from build123d import *

# Parameters (mm, degrees)
ESBO_O1_W                = 40
ESBO_O1_H                = 50
ESBO_O1_R                = 2
ESBO_O1_H_2              = 20
RESSALTO_EXTRUS_O1_DEPTH = 6
FILETE1_R                = 10


with BuildPart() as part:
    # Esboço1 → Ressalto-extrusão1 (new body)
    # profile 1 of 2: a face of its own
    with BuildSketch(Plane.XY):
        with Locations((20, 25)):
            Rectangle(ESBO_O1_W, ESBO_O1_H)
        with Locations((30, 10)):
            Circle(ESBO_O1_R, mode=Mode.SUBTRACT)
        with Locations((10, 10)):
            Circle(ESBO_O1_R, mode=Mode.SUBTRACT)
        with Locations((30, 40)):
            Circle(ESBO_O1_R, mode=Mode.SUBTRACT)
        with Locations((10, 40)):
            Circle(ESBO_O1_R, mode=Mode.SUBTRACT)
    # profile 2 of 2: a face of its own
    with BuildSketch(Plane.XY):
        with Locations((60, 10)):
            Rectangle(ESBO_O1_W, ESBO_O1_H_2)
        with Locations((50, 10)):
            Circle(ESBO_O1_R, mode=Mode.SUBTRACT)
        with Locations((70, 10)):
            Circle(ESBO_O1_R, mode=Mode.SUBTRACT)
    extrude(amount=RESSALTO_EXTRUS_O1_DEPTH)

    # Filete1
    filete1_edges = [part.edges().sort_by_distance(p)[0] for p in [
        (40, 20, 3),
    ]]
    fillet(filete1_edges, radius=FILETE1_R)


solid = part.part
Verification items for the finished model (mm, model axes). A direction names the side the tool comes from. Coordinates: 2 decimals unless noted, no trailing zeros. Write each loop counter-clockwise with the first axis right and the second up, starting at its lowest first coordinate (ties: lowest second). Pieces come first, ordered by that corner, then holes. Notation, with made-up numbers: (88, -0.75) - (123, -0.75) arc R30 ccw to (123, 28.25) - close; hole circle Ø1 at (15.25, 24). An arc over 180 degrees is marked (long way). Answer as a JSON object with one key per item and string values.
(1) Cross-section at A-A on y = 10. Record the cut outline in (x, z).
Report:
{"outline": "(0, 0) - (8, 0) - (8, 6) - (0, 6) - close; (12, 0) - (28, 0) - (28, 6) - (12, 6) - close; (32, 0) - (48, 0) - (48, 6) - (32, 6) - close; (52, 0) - (68, 0) - (68, 6) - (52, 6) - close; (72, 0) - (80, 0) - (80, 6) - (72, 6) - close"}
(2) Cross-section at C-C on z = 2. Record the cut outline in (x, y).
Report:
{"outline": "(0, 0) - (80, 0) - (80, 20) - (50, 20) arc R10 cw to (40, 30) - (40, 50) - (0, 50) - close; hole circle Ø4 at (10, 10); hole circle Ø4 at (10, 40); hole circle Ø4 at (30, 10); hole circle Ø4 at (30, 40); hole circle Ø4 at (50, 10); hole circle Ø4 at (70, 10)"}
(3) Mould release check, pull along X, two halves, no side actions. Record for faces 3 (the cylindrical face through (71.908, 10.601, 2.958)), 4 (the flat face through (31, 20, 6)), 5 (the flat face through (40, 40, 3)): pulls with the +X half, pulls with the -X half, needs draft (parallel to the pull), parting line crosses it, or undercut.
Report:
{"face 3": "undercut", "face 4": "needs draft", "face 5": "pulls with the +X half"}
(4) Cross-section at B-B on x = 70. Record the cut outline in (y, z), plus the area to 3 significant figures.
Report:
{"outline": "(0, 0) - (8, 0) - (8, 6) - (0, 6) - close; (12, 0) - (20, 0) - (20, 6) - (12, 6) - close", "area": "96.0 mm^2"}
(5) Cross-section at D-D on x = 10. Record the cut outline in (y, z), plus the area to 3 significant figures.
Report:
{"outline": "(0, 0) - (8, 0) - (8, 6) - (0, 6) - close; (12, 0) - (38, 0) - (38, 6) - (12, 6) - close; (42, 0) - (50, 0) - (50, 6) - (42, 6) - close", "area": "252 mm^2"}
(6) Gauge pin test, flat ends, axial feed: pin 1 Ø2 at (y, z) = (34, 4) entering from +X; pin 2 Ø1.8 at (x, z) = (65.5, 3) entering from +Y. Record the tip position at first contact, or that the pin passes through.
Report:
{"pin 1": "x = 40", "pin 2": "y = 20"}
(7) Tool access check on faces 1 (the flat face through (65, 20, 3)), 2 (the flat face through (39, 0, 3)). Record the directions out of +Z, -Z, +X, -X, +Y, -Y that give a thin tool (end or side, any length) a straight path to the whole face; none if there is none.
Report:
{"face 1": "+Z, -Z, +X, +Y", "face 2": "+Z, -Z, +X, -X, -Y"}
(8) Thickness scan on line 1 along Y through (x, z) = (30, 3.35); line 2 along Y through (x, z) = (9.5, 1.25); line 3 along X through (y, z) = (42.5, 4.65). Record the ranges inside material, lowest first.
Report:
{"line 1": "0 to 8, 12 to 38, 42 to 50", "line 2": "0 to 8.06, 11.94 to 38.06, 41.94 to 50", "line 3": "0 to 40"}
